Source: CAD feature listing. Evaluate the final solid. Frame: model axes, mm. A direction names the side the tool comes from. Give positions to 0.01 mm unless a question says otherwise; leave off trailing zeros. Loops run counter-clockwise (first coordinate to the right, second up) from the corner with the lowest first, then second, coordinate; pieces in that order, holes last. Notation, with made-up numbers: (-4, 77) - (1, 77) arc R6 ccw to (1, 88) - close; hole circle Ø3 at (10, -3). An arc over 180 degrees is marked (long way). Write each question's results on one line, items separated by ' | '. Start each with the question number.
(1) Cut plane A-A on y = -61. Return the cut outline in (x, z).
(2) Reachability of faces 4 (the flat face through (-90.918, -25, 38)), 5 (the flat face through (-94.891, -39, -3)), 6 (the flat face through (-90.918, -39, 25)), 7 (the flat face through (-95.586, -85, -11)), 8 (the flat face through (-93, -39, 7)) from +Z, -Z, +X, -X, +Y, -Y: full face, straight path, thin tool, end or side. Return the list, or none.
(3) Cut plane B-B on x = -3. Return the cut outline in (y, z), then the cut area to 3 significant figures.
(4) Cut plane D-D on z = 9.5. Return the cut outline in (x, y), then the cut area to 3 significant figures.
(5) Pull-direction query (X, two-part tool) for faces 1 (the flat face through (-38, -39, 28)), 2 (the flat face through (16.109, -49, 15)), 3 (the cylindrical face through (-120.417, -48.041, 19.15)); classes: pulls with the +X half, pulls with the -X half, needs draft (parallel to the pull), parting line crosses it, or undercut.
(6) Cut plane C-C on y = -27. Return the cut outline in (x, z).
(7) Contact query for flat-ended pins moving along their axis: pin 1 (6.5 mm diameter, centred on x = -80.67, z = 14.25, fed in from -Y); pin 2 (1.4 mm diameter, centred on x = -123.42, z = 14.25, fed in from -Y) (1 decimal); pin 3 (2 mm diameter, centred on y = -101, z = 40.5, fed in from +X); pin 4 (13.5 mm diameter, centred on y = -25, z = 32, fed in from -X). Output: stop coordinate, or through.
(8) Material intervals for line 1 along X through (y, z) = (-22.2, -4.15); line 2 along X through (y, z) = (-47, 14); line 3 along Y through (x, z) = (-28, 29.5), sorted ascending. Write a range as [from, to].
from build123d import *

# Parameters (mm, degrees)
SKETCH4_W                  = 106
SKETCH4_H                  = 30
BOSS_EXTRUDE2_DEPTH        = 13
SKETCH25_W                 = 106
SKETCH25_H                 = 8.1
CUT_EXTRUDE3_DEPTH         = 1
CUT_EXTRUDE3_DEPTH_BACK    = 8.3
M3X0_5_TAPPED_HOLE1_D      = 2.5
SKETCH28_W                 = 106
SKETCH28_H                 = 4.5
BOSS_EXTRUDE3_DEPTH        = 41.5
SKETCH32_W                 = 41.5
SKETCH32_H                 = 4.5
BOSS_EXTRUDE10_DEPTH       = 5
SKETCH33_W                 = 13
SKETCH33_H                 = 17.621445937
BOSS_EXTRUDE12_DEPTH       = 5
SKETCH34_W                 = 4.498886861
SKETCH34_H                 = 13.121445937
BOSS_EXTRUDE13_DEPTH       = 7
SKETCH35_W                 = 54.5
SKETCH35_H                 = 4.5
BOSS_EXTRUDE14_DEPTH       = 40
SKETCH36_W                 = 5
SKETCH36_H                 = 20
BOSS_EXTRUDE15_DEPTH       = 13.12
F_8_0_199_DIAMETER_HOLE1_D = 5.0546
SKETCH39_R                 = 7
CUT_EXTRUDE4_DEPTH         = 10
M2_CLEARANCE_HOLE1_D       = 2.4
SKETCH43_W                 = 35.304815243
SKETCH43_H                 = 4
BOSS_EXTRUDE16_DEPTH       = 70
SKETCH44_W                 = 107.027081708
SKETCH44_H                 = 13.5
BOSS_EXTRUDE17_DEPTH       = 25.5
SKETCH47_W                 = 107.027081708
SKETCH47_H                 = 8.1
CUT_EXTRUDE5_DEPTH         = 8.3
M3X0_5_TAPPED_HOLE2_D      = 2.5


with BuildPart() as part:
    # Sketch4 → Boss-Extrude2 (new body)
    with BuildSketch(Plane.XY):
        with Locations((-36.891047602, -35.322762913)):
            Rectangle(SKETCH4_W, SKETCH4_H)
    extrude(amount=-BOSS_EXTRUDE2_DEPTH)

    # Sketch25 → Cut-Extrude3 (cut, two sides)
    with BuildSketch(Plane.XY) as cut_extrude3_sk:
        with Locations((-36.891047602, -28.651316976)):
            Rectangle(SKETCH25_W, SKETCH25_H)
    extrude(amount=CUT_EXTRUDE3_DEPTH, mode=Mode.SUBTRACT)
    extrude(cut_extrude3_sk.sketch, amount=-CUT_EXTRUDE3_DEPTH_BACK, mode=Mode.SUBTRACT)

    # M3x0.5 Tapped Hole1 (through all)
    with Locations(Plane(origin=(-74.390985602, -20.322762913, -4.15), x_dir=(0, 0, 1), z_dir=(0, 1, 0))):
        with Locations((0, 0), (0, 25), (-0.055677319, 74.999938), (0, 50)):
            Hole(M3X0_5_TAPPED_HOLE1_D / 2)

    # Sketch28 → Boss-Extrude3 (add)
    with BuildSketch(Plane.XY):
        with Locations((-36.891047602, -48.072762913)):
            Rectangle(SKETCH28_W, SKETCH28_H)
    extrude(amount=BOSS_EXTRUDE3_DEPTH)

    # Sketch32 → Boss-Extrude10 (add)
    with BuildSketch(Plane.ZY.offset(89.891047602)):
        with Locations((20.75, -48.072762913)):
            Rectangle(SKETCH32_W, SKETCH32_H)
    extrude(amount=BOSS_EXTRUDE10_DEPTH)

    # Sketch33 → Boss-Extrude12 (add)
    with BuildSketch(Plane.ZY.offset(89.891047602)):
        with Locations((-6.5, -41.512039945)):
            Rectangle(SKETCH33_W, SKETCH33_H)
    extrude(amount=BOSS_EXTRUDE12_DEPTH)

    # Sketch34 → Boss-Extrude13 (add)
    with BuildSketch(Plane.XY):
        with Locations((-92.641604172, -39.262039945)):
            Rectangle(SKETCH34_W, SKETCH34_H)
    extrude(amount=BOSS_EXTRUDE13_DEPTH)

    # Sketch35 → Boss-Extrude14 (add)
    with BuildSketch(Plane.ZY.offset(94.891047602)):
        with Locations((14.25, -48.072762913)):
            Rectangle(SKETCH35_W, SKETCH35_H)
    extrude(amount=BOSS_EXTRUDE14_DEPTH)

    # Sketch36 → Boss-Extrude15 (add)
    with BuildSketch(Plane(origin=(0, -45.822762913, 0), x_dir=(1, 0, 0), z_dir=(0, 1, 0))):
        with Locations((-93.41812931, -31.5)):
            Rectangle(SKETCH36_W, SKETCH36_H)
    extrude(amount=BOSS_EXTRUDE15_DEPTH)

    # #8 (0.199) Diameter Hole1 (through all)
    with Locations(Plane(origin=(-80.669073904, -45.822762913, 14.25), x_dir=(0, 0, 1), z_dir=(0, 1, 0))):
        with Locations((0, 0), (0, 91.778026302), (0, 81.778026302), (0, 10)):
            Hole(F_8_0_199_DIAMETER_HOLE1_D / 2)

    # Sketch39 → Cut-Extrude4 (cut)
    with BuildSketch(Plane(origin=(0, -45.822762913, 0), x_dir=(1, 0, 0), z_dir=(0, 1, 0))):
        with Locations((-115.41812931, -14.25)):
            Circle(SKETCH39_R)
    extrude(amount=-CUT_EXTRUDE4_DEPTH, mode=Mode.SUBTRACT)

    # M2 Clearance Hole1 (through all)
    with Locations(Plane(origin=(-107.41812931, -45.822762913, 14.25), x_dir=(0, 0, 1), z_dir=(0, 1, 0))):
        with Locations((0, 0), (8.000007036, -8.002918292), (-7.999992964, -8.002918292), (0, -16)):
            Hole(M2_CLEARANCE_HOLE1_D / 2)

    # Sketch43 → Boss-Extrude16 (add)
    with BuildSketch(Plane(origin=(0, -50.322762913, 0), x_dir=(-1, 0, 0), z_dir=(0, -1, 0))):
        Polygon((95.586232359, -37.5), (95.586232359, -41.5), (134.891047602, -41.5), (134.891047602, -37.5), (130.891047602, -37.5), align=None)
        Polygon((130.891047602, -37.5), (134.891047602, -37.5), (134.891047602, 13), (130.891047602, 13), (130.891047602, 9), align=None)
        with Locations((113.238639981, 11)):
            Rectangle(SKETCH43_W, SKETCH43_H)
    extrude(amount=BOSS_EXTRUDE16_DEPTH)

    # Sketch44 → Boss-Extrude17 (add)
    with BuildSketch(Plane(origin=(0, -45.822762913, 0), x_dir=(1, 0, 0), z_dir=(0, 1, 0))):
        with Locations((-37.404588456, -34.75)):
            Rectangle(SKETCH44_W, SKETCH44_H)
    extrude(amount=BOSS_EXTRUDE17_DEPTH)

    # Sketch47 → Cut-Extrude5 (cut)
    with BuildSketch(Plane(origin=(0, 0, 28), x_dir=(-1, 0, 0), z_dir=(0, 0, -1))):
        with Locations((37.404588456, -28.652762913)):
            Rectangle(SKETCH47_W, SKETCH47_H)
    extrude(amount=-CUT_EXTRUDE5_DEPTH, mode=Mode.SUBTRACT)

    # M3x0.5 Tapped Hole2 (through all)
    with Locations(Plane(origin=(-74.391047602, -20.322762913, 32.71), x_dir=(0, 0, 1), z_dir=(0, 1, 0))):
        with Locations((0, 0), (0, 25), (0, 50), (0, 75)):
            Hole(M3X0_5_TAPPED_HOLE2_D / 2)


solid = part.part
Ans:
1) outline: (-134.89, -13) - (-95.59, -13) - (-95.59, -9) - (-130.89, -9) - (-130.89, 37.5) - (-95.59, 37.5) - (-95.59, 41.5) - (-134.89, 41.5) - close
2) face 4: +Z, -Z, -X, +Y | face 5: -Z, -X, +Y | face 6: +X, +Y | face 7: +Z, -Z, +X, -Y | face 8: +X, -X, +Y
3) outline: (-50.32, -13) - (-20.32, -13) - (-20.32, 0) - (-24.6, 0) - (-24.6, -8.3) - (-32.7, -8.3) - (-32.7, 0) - (-45.82, 0) - (-45.82, 28) - (-32.7, 28) - (-32.7, 36.3) - (-24.6, 36.3) - (-24.6, 28) - (-20.32, 28) - (-20.32, 41.5) - (-50.32, 41.5) - close | area: 787 mm^2
4) outline: (-134.89, -120.32) - (-130.89, -120.32) - (-130.89, -50.32) - (-120.56, -50.32) - (-120.56, -45.82) - (-134.89, -45.82) - close; (-110.28, -50.32) - (16.11, -50.32) - (16.11, -45.82) - (-110.28, -45.82) - close | area: 913 mm^2
5) face 1: needs draft | face 2: pulls with the +X half | face 3: undercut
6) outline: (-90.92, 36.3) - (16.11, 36.3) - (16.11, 41.5) - (-90.92, 41.5) - close; (-89.89, -13) - (16.11, -13) - (16.11, -8.3) - (-89.89, -8.3) - close
7) pin 1: y = -50.32 | pin 2: through | pin 3: x = -95.59 | pin 4: x = -90.92
8) line 1: [-89.89, -75.64], [-73.14, -50.64], [-48.14, -25.64], [-23.14, -0.64], [1.86, 16.11] | line 2: [-134.89, -124.59], [-106.24, -83.18], [-78.15, -73.18], [-68.15, -1.41], [3.62, 8.59], [13.62, 16.11] | line 3: [-50.32, -32.7], [-24.6, -20.32]
